Autodesk Inventor part; units mm, degrees
ref_plane "YZ Plane" through (0, 0, 0) normal (1, 0, 0) x (0, 1, 0)
ref_plane "XZ Plane" through (0, 0, 0) normal (0, 1, 0) x (-1, 0, 0)
ref_plane "XY Plane" through (0, 0, 0) normal (0, 0, 1) x (1, 0, 0)
ref_plane "РабПлоскость1" through (0, 0, 0) normal (0, 0, 1) x (1, 0, 0)
sketch "Эскиз1" plane through (0, 0, 0) normal (0, 0, 1) x (1, 0, 0)
  line L0 (45.389, -67.917) -> (45.389, 67.917)
  line L1 (45.389, 67.917) -> (-45.389, 67.917)
  line L2 (-45.389, -67.917) -> (45.389, -67.917)
  line L3 (-45.389, 67.917) -> (-45.389, -67.917)
  line L4 (41.8047, 51.1354) -> (28.1516, 51.1354)
  line L5 (28.1516, 51.1354) -> (28.1516, 31.897)
  line L6 (28.1516, 31.897) -> (41.8047, 31.897)
  line L7 (41.8047, 31.897) -> (41.8047, 51.1354)
  circle A0 centre (36.389, 27.7057) radius 2.75
  circle A1 centre (0, -60.917) radius 2.75
  circle A2 centre (-36.389, 27.7057) radius 2.75
  circle A3 centre (36.389, 27.7057) radius 2
  circle A4 centre (0, -60.917) radius 2
  circle A5 centre (-36.389, 27.7057) radius 2
  point P0 (0, 0)
extrude "Выдавливание1" add sketch "Эскиз1" along normal blind 3 contours L2 L3 L1 L0 | A0 | A1 | A2
sketch "Эскиз2" plane through (0, 0, 0) normal (0, 0, -1) x (-1, 0, 0)
  line L0 (42.389, -64.917) -> (-42.389, -64.917)
  line L1 (-42.389, -64.917) -> (-42.389, 54.5577)
  line L2 (-42.611, 64.083) -> (10.389, 64.083)
  line L3 (42.389, 64.917) -> (42.389, -64.917)
  line L4 (-32.389, -64.917) -> (-12.389, -64.917)
  line L5 (-12.389, -64.917) -> (-12.389, -62.917)
  line L6 (-12.389, -62.917) -> (-32.389, -62.917)
  line L7 (-32.389, -62.917) -> (-32.389, -64.917)
  line L8 (-32.389, 64.083) -> (-12.389, 64.083)
  line L9 (-12.389, 64.083) -> (-12.389, 62.083)
  line L10 (-12.389, 62.083) -> (-32.389, 62.083)
  line L11 (-32.389, 62.083) -> (-32.389, 64.083)
  line L12 (-32.389, 62.083) -> (-12.389, 62.083)
  line L13 (-12.389, 62.083) -> (-12.389, 60.083)
  line L14 (-12.389, 60.083) -> (-32.389, 60.083)
  line L15 (-32.389, 60.083) -> (-32.389, 62.083)
  line L16 (42.389, -10) -> (40.389, -10)
  line L17 (40.389, -10) -> (40.389, 10)
  line L18 (40.389, 10) -> (42.389, 10)
  line L19 (42.389, 10) -> (42.389, -10)
  point P0 (0, 0)
  point P1 (-12.389, 64.083)
  dimension "d5" = 20
  dimension "d6" = 10
  dimension "d7" = 2
  dimension "d8" = 2
  dimension "d9" = 2
  dimension "d10" = 2
  dimension "d11" = 20
  dimension "d12" = 10
extrude "Выдавливание2" add sketch "Эскиз2" along normal blind 2 contours L0 L7 L6 L5 | L16 L17 L18 L3 | L2 L9 L10 L11
sketch "Эскиз3" plane through (0, 0, 3) normal (0, 0, 1) x (1, 0, 0)
  circle A0 centre (-6.389, 60.583) radius 2.75
  circle A1 centre (-6.389, 35.583) radius 2.75
  point P0 (0, 0)
extrude "Выдавливание3" cut sketch "Эскиз3" against normal blind 2
sketch "Эскиз4" plane through (0, 0, 3) normal (0, 0, 1) x (1, 0, 0)
  line L0 (-33.889, -18.417) -> (41.111, -18.417)
  circle A0 centre (-6.389, 35.583) radius 2.75
  circle A1 centre (-6.389, 60.583) radius 2.75
  line L1 (45.389, 67.917) -> (-45.389, 67.917)
  line L2 (-45.389, 67.917) -> (-45.389, -67.917)
  line L3 (-45.389, -67.917) -> (45.389, -67.917)
  line L4 (45.389, -67.917) -> (45.389, 67.917)
  circle A2 centre (36.389, 27.7057) radius 2
  circle A3 centre (0, -60.917) radius 2
  circle A4 centre (-36.389, 27.7057) radius 2
  line L5 (41.8047, 51.1354) -> (41.8047, 31.897)
  line L6 (41.8047, 31.897) -> (28.1516, 31.897)
  line L7 (28.1516, 31.897) -> (28.1516, 51.1354)
  line L8 (28.1516, 51.1354) -> (41.8047, 51.1354)
  point P0 (0, 0)
extrude "Выдавливание4" add sketch "Эскиз4" along normal blind 1
equation "\"d9\" = d8"
properties part number "top"
Geometry check sheet. Reference: the model listing, model coordinates, mm. A direction names the side the tool comes from. Give positions to 0.01 mm unless a question says otherwise; leave off trailing zeros. Order: outer loops, then holes, each group sorted by start corner. A loop starts at its lowest first (then second) coordinate and runs counter-clockwise, first axis right, second up.
1. Gauge pin test, flat ends, axial feed: pin 1 Ø1 at (x, y) = (-2, 5.5) entering from -Z; pin 2 Ø0.6 at (x, z) = (21, -1) entering from -Y; pin 3 Ø1.6 at (x, y) = (-6, 37) entering from +Z. Record the tip position at first contact, or that the pin passes through.
2. Section check C-C, the plane x = 22.5. Enter the section's corners in (y, z).
3. Section check D-D, the plane x = 36.5. Enter the section's corners in (y, z).
4. Release check for a two-part mould opening along X. For faces 1 (the face through (45.389, -1, 2)), 2 (the face through (-1, -67.917, 2)), 3 (the face through (-6.985, 63.268, 2.479)), 4 (the face through (-45.389, 1, 2)) record: pulls with the +X half, pulls with the -X half, needs draft (parallel to the pull), parting line crosses it, or undercut.
5. Thickness scan on L1, parallel to Y at x = 0, z = 2.45; L2, parallel to Y at x = 29, z = 2.65; L3, parallel to Y at x = -8, z = 3. Record the ranges inside material, lowest first.
6. Section check A-A, the plane x = 0. Enter the section's corners in (y, z).
7. Access from +Z, -Z, +X, -X, +Y, -Y to the whole of each face (thin tool, end or side, straight path). Record for faces 5 (the face through (-6, 61, 1)), 6 (the face through (28.152, 41, 2)), 7 (the face through (1, 67.917, 2)).
8. Section check B-B, the plane y = 49.5. Enter the section's corners in (x, z).
Values follow:
1. pin 1: stops at z = 0
1. pin 2: stops at y = -64.92
1. pin 3: stops at z = 1
2. outline: (-67.92, 0) - (-64.92, 0) - (-64.92, -2) - (-62.92, -2) - (-62.92, 0) - (62.08, 0) - (62.08, -2) - (64.08, -2) - (64.08, 0) - (67.92, 0) - (67.92, 4) - (-67.92, 4) - close
3. outline: (-67.92, 0) - (25.71, 0) - (25.71, 4) - (-67.92, 4) - close; (29.7, 0) - (31.9, 0) - (31.9, 4) - (29.7, 4) - close; (51.14, 0) - (67.92, 0) - (67.92, 4) - (51.14, 4) - close
4. face 1: pulls with the +X half
4. face 2: needs draft
4. face 3: undercut
4. face 4: pulls with the -X half
5. L1: y = -67.92 to -62.92, -58.92 to 67.92
5. L2: y = -67.92 to 31.9, 51.14 to 67.92
5. L3: y = -67.92 to 33.35, 37.81 to 58.35, 62.81 to 67.92
6. outline: (-67.92, 0) - (-62.92, 0) - (-62.92, 4) - (-67.92, 4) - close; (-58.92, 0) - (67.92, 0) - (67.92, 4) - (-58.92, 4) - close
7. face 5: +Z
7. face 6: +Z, -Z
7. face 7: +Z, -Z, +X, -X, +Y
8. outline: (-45.39, 0) - (28.15, 0) - (28.15, 4) - (-45.39, 4) - close; (41.8, 0) - (45.39, 0) - (45.39, 4) - (41.8, 4) - close
